Answer from the drawing. Dimensions are ordinates in mm from the lowest x, y and z of the part. Coordinates: 2 decimals unless noted, no trailing zeros. Write each loop counter-clockwise with the first axis right and the second up, starting at its lowest first coordinate (ties: lowest second). Pieces come first, ordered by that corner, then holes.
(1) Section C-C on x = 159 is taken. Write down the section's boundary in (y, z), then the cut area to 3 significant figures.
(2) Section B-B on y = 23 is taken. Write down the section's boundary in (x, z).
(3) Section A-A on z = 4.25 is taken. Write down the section's boundary in (x, y).
(4) Given pin 1 (3 mm diameter, centred on y = 23, z = 3, fed in from +X); pin 2 (3 mm diameter, centred on x = 173, z = 2.5, fed in from -Y); pin 3 (3 mm diameter, centred on x = 18, z = 4, fed in from +Y), each flat-ended and moving along its own axis, determine where each tip first touches the part or whether it passes through.
(5) Find the intervals of material crossed by probe 1 along X at (y, z) = (22, 4.25); probe 2 along Y at (x, z) = (30.5, 3.75), in increasing order.
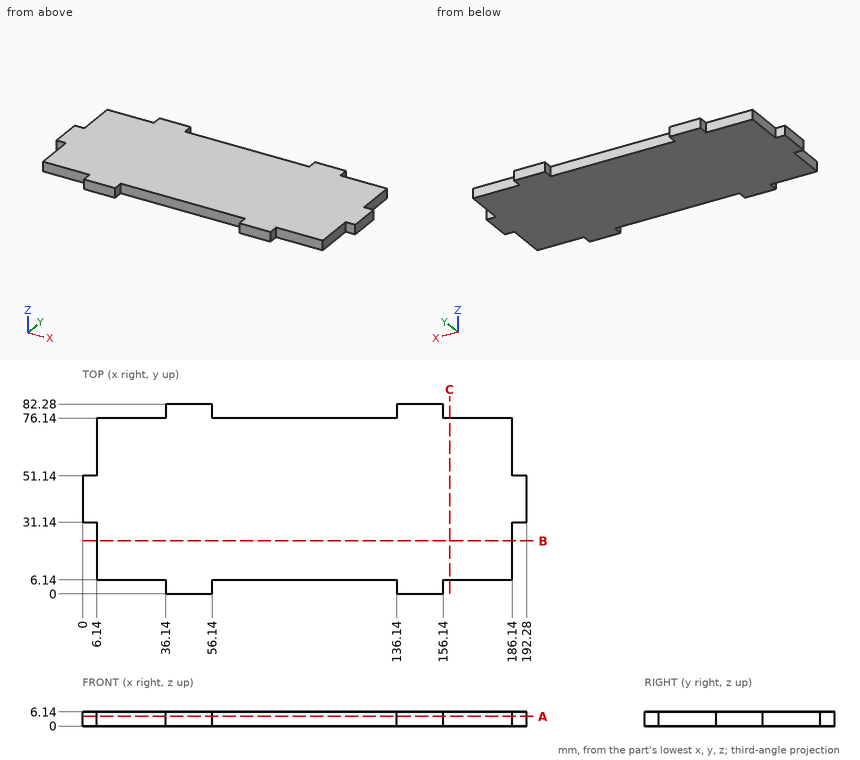
Response:
1. outline: (6.14, 0) - (76.14, 0) - (76.14, 6.14) - (6.14, 6.14) - close
1. area: 430 mm2
2. outline: (6.14, 0) - (186.14, 0) - (186.14, 6.14) - (6.14, 6.14) - close
3. outline: (0, 31.14) - (6.14, 31.14) - (6.14, 6.14) - (36.14, 6.14) - (36.14, 0) - (56.14, 0) - (56.14, 6.14) - (136.14, 6.14) - (136.14, 0) - (156.14, 0) - (156.14, 6.14) - (186.14, 6.14) - (186.14, 31.14) - (192.28, 31.14) - (192.28, 51.14) - (186.14, 51.14) - (186.14, 76.14) - (156.14, 76.14) - (156.14, 82.28) - (136.14, 82.28) - (136.14, 76.14) - (56.14, 76.14) - (56.14, 82.28) - (36.14, 82.28) - (36.14, 76.14) - (6.14, 76.14) - (6.14, 51.14) - (0, 51.14) - close
4. pin 1: stops at x = 186.14
4. pin 2: stops at y = 6.14
4. pin 3: stops at y = 76.14
5. probe 1: x = 6.14 to 186.14
5. probe 2: y = 6.14 to 76.14
